```python
from build123d import *

# Parameters (mm, degrees)
SKETCH_1_W          = 15
SKETCH_1_H          = 15
SKETCH_1_W_2        = 13
SKETCH_1_H_2        = 13
EXTRUDE_1_DEPTH     = 125
SKETCH_2_R          = 1.6
CUT_EXTRUDE_1_DEPTH = 127.787223331
SKETCH_3_R          = 1.6
CUT_EXTRUDE_2_DEPTH = 127.787223331


with BuildPart() as part:
    # 草图1 → 拉伸-薄壁1 (new body)
    with BuildSketch(Plane.XY):
        with Locations((7.5, -7.5)):
            Rectangle(SKETCH_1_W, SKETCH_1_H)
        with Locations((7.5, -7.5)):
            Rectangle(SKETCH_1_W_2, SKETCH_1_H_2, mode=Mode.SUBTRACT)
    extrude(amount=EXTRUDE_1_DEPTH)

    # 草图2 → 切除-拉伸1 (cut, through all)
    with BuildSketch(Plane(origin=(15, 0, 0), x_dir=(0, 0, -1), z_dir=(1, 0, 0))):
        with Locations((-105, -3.75)):
            Circle(SKETCH_2_R)
        with Locations((-105, -11.25)):
            Circle(SKETCH_2_R)
        with Locations((-95, -11.25)):
            Circle(SKETCH_2_R)
        with Locations((-95, -3.75)):
            Circle(SKETCH_2_R)
        with Locations((-22.5, -3.75)):
            Circle(SKETCH_2_R)
        with Locations((-22.5, -11.25)):
            Circle(SKETCH_2_R)
        with Locations((-32.5, -11.25)):
            Circle(SKETCH_2_R)
        with Locations((-32.5, -3.75)):
            Circle(SKETCH_2_R)
        with Locations((-57.5, -11.25)):
            Circle(SKETCH_2_R)
        with Locations((-67.5, -11.25)):
            Circle(SKETCH_2_R)
        with Locations((-67.5, -3.75)):
            Circle(SKETCH_2_R)
        with Locations((-57.5, -3.75)):
            Circle(SKETCH_2_R)
        Polygon((-87, -2), (-87, -13), (-78, -13), align=None)
        Polygon((-82.5, -2), (-73.5, -2), (-73.5, -13), align=None)
        Polygon((-51.5, -13), (-42.5, -2), (-51.5, -2), align=None)
        Polygon((-47, -13), (-38, -2), (-38, -13), align=None)
    extrude(amount=-CUT_EXTRUDE_1_DEPTH, mode=Mode.SUBTRACT)

    # 草图3 → 切除-拉伸2 (cut, through all)
    with BuildSketch(Plane(origin=(0, 0, 0), x_dir=(1, 0, 0), z_dir=(0, 1, 0))):
        with Locations(Location((3.75, -5, 0), (0, 0, 270))):
            Circle(SKETCH_3_R)
        with Locations(Location((11.25, -5, 0), (0, 0, 90))):
            Circle(SKETCH_3_R)
        with Locations(Location((11.25, -15, 0), (0, 0, 270))):
            Circle(SKETCH_3_R)
        with Locations(Location((3.75, -15, 0), (0, 0, 90))):
            Circle(SKETCH_3_R)
        with Locations(Location((3.75, -57.5, 0), (0, 0, 270))):
            Circle(SKETCH_3_R)
        with Locations(Location((11.25, -57.5, 0), (0, 0, 90))):
            Circle(SKETCH_3_R)
        with Locations(Location((11.25, -67.5, 0), (0, 0, 270))):
            Circle(SKETCH_3_R)
        with Locations(Location((3.75, -67.5, 0), (0, 0, 90))):
            Circle(SKETCH_3_R)
        with Locations(Location((3.75, -110, 0), (0, 0, 270))):
            Circle(SKETCH_3_R)
        with Locations(Location((11.25, -110, 0), (0, 0, 90))):
            Circle(SKETCH_3_R)
        with Locations(Location((11.25, -120, 0), (0, 0, 270))):
            Circle(SKETCH_3_R)
        with Locations(Location((3.75, -120, 0), (0, 0, 90))):
            Circle(SKETCH_3_R)
        Polygon((2.5, -25), (2.5, -31), (12.5, -31), align=None)
        Polygon((2.5, -22), (12.5, -22), (12.5, -28), align=None)
        Polygon((2.5, -37), (12.5, -37), (12.5, -43), align=None)
        Polygon((12.5, -46), (2.5, -40), (2.5, -46), align=None)
        Polygon((2.5, -79), (12.5, -79), (2.5, -85), align=None)
        Polygon((12.5, -82), (2.5, -88), (12.5, -88), align=None)
        Polygon((12.5, -97), (2.5, -103), (12.5, -103), align=None)
        Polygon((12.5, -94), (2.5, -100), (2.5, -94), align=None)
    extrude(amount=-CUT_EXTRUDE_2_DEPTH, mode=Mode.SUBTRACT)


solid = part.part
```
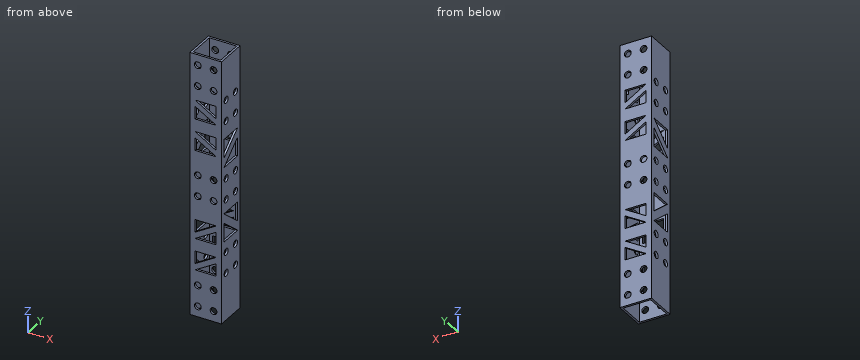
The model under review builds one solid part; all positions refer to its coordinate system, in mm. Round coordinates to 2 decimals unless told otherwise and drop trailing zeros. Order: outer loops, then holes, each group sorted by start corner. A loop starts at its lowest first (then second) coordinate and runs counter-clockwise, first axis right, second up. Notation, with made-up numbers: (-26, 40) -> (7, 40) arc R15 ccw to (7, 64) -> close; hole circle Ø10 at (-28, 37). An arc over 180 degrees is marked (long way). One line per item, written item: value. Start each with the question number.
Q1. Take a section at B-B (z = 63). Write out the cut boundary in (x, y).
Q2. Wall thickness on line 1 (X direction, y = -0.25, z = 15); line 2 (Y direction, x = 14.8, z = 105); line 3 (X direction, y = -11.5, z = 110.5): over which ranges is each line inside the solid? List them lowest first.
Q3. Take a section at C-C (x = 7.5). Count the separate pieces of the cut face and the enclosed holes in it, and give its area (3 significant figures).
Q4. Take a section at A-A (z = 15). Write out the cut boundary in (x, y).
Reported:
1. outline: (0, -15) -> (15, -15) -> (15, 0) -> (0, 0) -> close; hole (1, -14) -> (14, -14) -> (14, -1) -> (1, -1) -> close
2. line 1: x = 0 to 2.15, 5.35 to 9.65, 12.85 to 15
2. line 2: y = -15 to -12.85, -9.65 to -5.35, -2.15 to 0
2. line 3: x = 0 to 1, 14 to 15
3. separate pieces: 18
3. enclosed holes: 0
3. area: 202 mm2
4. outline: (0, -15) -> (2.15, -15) -> (2.15, -14) -> (1, -14) -> (1, -1) -> (2.15, -1) -> (2.15, 0) -> (0, 0) -> close; (5.35, -15) -> (9.65, -15) -> (9.65, -14) -> (5.35, -14) -> close; (5.35, -1) -> (9.65, -1) -> (9.65, 0) -> (5.35, 0) -> close; (12.85, -15) -> (15, -15) -> (15, 0) -> (12.85, 0) -> (12.85, -1) -> (14, -1) -> (14, -14) -> (12.85, -14) -> close
